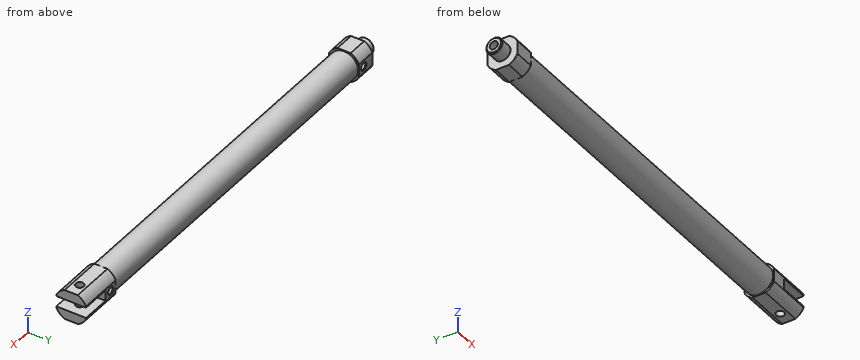
Autodesk Inventor part; units mm, degrees
ref_plane "BODY_N_XY" through (257, 0, 0) normal (0, 0, -1) x (1, 0, 0)
ref_plane "BODY_N_YZ" through (257, 0, 0) normal (1, 0, 0) x (0, -1, 0)
ref_plane "BODY_N_ZX" through (257, 0, 0) normal (0, -1, 0) x (0, 0, -1)
sketch "Sketch_8" plane through (0, 0, 0) normal (0, 0, 1) x (1, 0, 0)
  line L0 (0, 0) -> (-8, 0)
  line L1 (-8, 0) -> (-8, 4.3865)
  line L2 (-8, 4.3865) -> (-7.3865, 5)
  line L3 (-7.3865, 5) -> (0, 5)
  line L4 (0, 5) -> (0, 0)
  line L5 (0, 0) -> (-8, 0)
revolve "Revolution1" add sketch "Sketch_8" angle 360 about axis through (0, 0, 0) along (1, 0, 0)
thread "Thread1"
sketch "Sketch_9" plane through (0, 0, 0) normal (1, 0, 0) x (0, 0, -1)
  line L0 (-9.15, 4.0345) -> (-9.15, -4.0345)
  arc A0 (-9.15, -4.0345) -> (-4.0345, -9.15) centre (0, 0) ccw
  line L1 (-4.0345, -9.15) -> (4.0345, -9.15)
  arc A1 (4.0345, -9.15) -> (9.15, -4.0345) centre (0, 0) ccw
  line L2 (9.15, -4.0345) -> (9.15, 4.0345)
  arc A2 (9.15, 4.0345) -> (4.0345, 9.15) centre (0, 0) ccw
  line L3 (4.0345, 9.15) -> (-4.0345, 9.15)
  arc A3 (-4.0345, 9.15) -> (-9.15, 4.0345) centre (0, 0) ccw
extrude "Extrusion1" add sketch "Sketch_9" along normal blind 12.5
sketch "Sketch_11" plane through (12.5, 0, 0) normal (1, 0, 0) x (0, 0, -1)
  circle A0 centre (0, 0) radius 8.7
extrude "Extrusion2" add sketch "Sketch_11" along normal blind 225
sketch "Sketch_10" plane through (237.5, 0, 0) normal (1, 0, 0) x (0, 0, -1)
  line L0 (-9.15, 4.0345) -> (-9.15, -4.0345)
  arc A0 (-9.15, -4.0345) -> (-4.0345, -9.15) centre (0, 0) ccw
  line L1 (-4.0345, -9.15) -> (4.0345, -9.15)
  arc A1 (4.0345, -9.15) -> (9.15, -4.0345) centre (0, 0) ccw
  line L2 (9.15, -4.0345) -> (9.15, 4.0345)
  arc A2 (9.15, 4.0345) -> (4.0345, 9.15) centre (0, 0) ccw
  line L3 (4.0345, 9.15) -> (-4.0345, 9.15)
  arc A3 (-4.0345, 9.15) -> (-9.15, 4.0345) centre (0, 0) ccw
extrude "Extrusion3" add sketch "Sketch_10" along normal blind 27.5
sketch "Sketch7" plane through (0, 0, 0) normal (0, 0, 1) x (1, 0, 0)
  line L0 (8, 9.15) -> (8, 4.15)
  line L1 (8, 2.9566) -> (5.933, 4.15)
  line L2 (5.933, 4.15) -> (5.933, 8.717)
  line L3 (5.933, 8.717) -> (5.5, 9.15)
  line L4 (5.5, 9.15) -> (8, 9.15)
  line L5 (8, 9.15) -> (8, 2.9566)
revolve "Revolution2" cut sketch "Sketch7" angle 360 about axis through (8, 9.15, 0) along (0, 1, 0)
thread "Thread2"
sketch "Sketch_7" plane through (0, 0, 0) normal (0, 0, 1) x (1, 0, 0)
  line L0 (242, 9.15) -> (242, 4.15)
  line L1 (242, 2.9566) -> (239.933, 4.15)
  line L2 (239.933, 4.15) -> (239.933, 8.717)
  line L3 (239.933, 8.717) -> (239.5, 9.15)
  line L4 (239.5, 9.15) -> (242, 9.15)
  line L5 (242, 9.15) -> (242, 2.9566)
revolve "Revolution3" cut sketch "Sketch_7" angle 360 about axis through (242, 9.15, 0) along (0, 1, 0)
thread "Thread3"
sketch "Sketch_16" plane through (0, 0, 0) normal (0, 0, 1) x (1, 0, 0)
  line L0 (217.5, 0) -> (-8, 0)
  line L1 (-8, 0) -> (-8, 2.5)
  line L2 (-8, 2.5) -> (12.5, 2.5)
  line L3 (12.5, 2.5) -> (12.5, 8)
  line L4 (12.5, 8) -> (217.5, 8)
  line L5 (217.5, 8) -> (217.5, 0)
  line L6 (217.5, 0) -> (-8, 0)
revolve "Revolution4" cut sketch "Sketch_16" angle 360 about axis through (217.5, 0, 0) along (1, 0, 0)
sketch "Sketch_3" plane through (0, 0, 0) normal (0, 1, 0) x (-1, 0, 0)
  line L0 (-247, 3.25) -> (-265, 3.25)
  line L1 (-265, 3.25) -> (-265, -3.25)
  line L2 (-265, -3.25) -> (-247, -3.25)
  line L3 (-247, -3.25) -> (-247, 3.25)
extrude "Extrusion4" cut sketch "Sketch_3" along normal mid plane 18.3
sketch "Sketch_13" plane through (0, 0, 0) normal (0, 0, 1) x (1, 0, 0)
  circle A0 centre (257, 0) radius 2.5
extrude "Extrusion5" cut sketch "Sketch_13" along normal mid plane 18.3
ref_plane "BODY_N_XY" through (257, 0, 0) normal (0, 0, -1) x (1, 0, 0)
ref_plane "BODY_N_YZ" through (257, 0, 0) normal (1, 0, 0) x (0, -1, 0)
ref_plane "BODY_N_ZX" through (257, 0, 0) normal (0, -1, 0) x (0, 0, -1)
ref_plane "BODY_PIN_XY" through (257, 0, 0) normal (-1, 0, 0) x (0, 0, -1)
ref_plane "BODY_PIN_YZ" through (257, 0, 0) normal (0, 0, -1) x (0, -1, 0)
ref_plane "BODY_PIN_ZX" through (257, 0, 0) normal (0, -1, 0) x (-1, 0, 0)
ref_plane "NUT2_XY" through (247, 0, 0) normal (1, 0, 0) x (0, 0, -1)
ref_plane "NUT2_YZ" through (247, 0, 0) normal (0, 0, -1) x (0, 1, 0)
ref_plane "NUT2_ZX" through (247, 0, 0) normal (0, 1, 0) x (1, 0, 0)
ref_plane "SW1_XY" through (17.5, 0, 0) normal (1, 0, 0) x (0, 0, -1)
ref_plane "SW1_YZ" through (17.5, 0, 0) normal (0, 0, -1) x (0, 1, 0)
ref_plane "SW1_ZX" through (17.5, 0, 0) normal (0, 1, 0) x (1, 0, 0)
ref_plane "SW2_XY" through (232.5, 0, 0) normal (-1, 0, 0) x (0, 0, -1)
ref_plane "SW2_YZ" through (232.5, 0, 0) normal (0, 0, -1) x (0, -1, 0)
ref_plane "SW2_ZX" through (232.5, 0, 0) normal (0, -1, 0) x (-1, 0, 0)
ref_plane "SW_R1_XY" through (17.5, -14.15, 0) normal (1, 0, 0) x (0, 0, -1)
ref_plane "SW_R1_YZ" through (17.5, -14.15, 0) normal (0, 0, -1) x (0, 1, 0)
ref_plane "SW_R1_ZX" through (17.5, -14.15, 0) normal (0, 1, 0) x (1, 0, 0)
ref_plane "SW_R2_XY" through (232.5, -14.15, 0) normal (-1, 0, 0) x (0, 0, -1)
ref_plane "SW_R2_YZ" through (232.5, -14.15, 0) normal (0, 0, -1) x (0, -1, 0)
ref_plane "SW_R2_ZX" through (232.5, -14.15, 0) normal (0, -1, 0) x (-1, 0, 0)
ref_plane "body_XY" through (0, 0, 0) normal (1, 0, 0) x (0, 0, -1)
ref_plane "body_YZ" through (0, 0, 0) normal (0, 0, -1) x (0, 1, 0)
ref_plane "body_ZX" through (0, 0, 0) normal (0, 1, 0) x (1, 0, 0)
properties part number "CJ2D16-200Z(1_0)_BODY"
Geometry check sheet. Reference: the model listing, model coordinates, mm. Round coordinates to 2 decimals unless told otherwise and drop trailing zeros. Loops run counter-clockwise (first coordinate to the right, second up) from the corner with the lowest first, then second, coordinate; pieces in that order, holes last. Notation, with made-up numbers: (43.5, 26) -> (89.5, 26) arc R7 cw to (89.5, 37) -> close; hole circle Ø3 at (-4, 52.25). An arc over 180 degrees is marked (long way). Answer as a JSON object with one key per item and string values. Group by question number.
Item 1: Thickness scan on line 1 along X through (y, z) = (2.5, 2.5); line 2 along X through (y, z) = (-5, 7.5); line 3 along X through (y, z) = (2, 4.5). Record the ranges inside material, lowest first.
Item 2: Cross-section at A-A, the plane x = 257. Record the cut outline in (y, z), plus the area to 3 significant figures.
Item 3: Depth check by flat-ended pin: pin 1 Ø6 at (x, z) = (131, -5.5) entering from -Y; pin 2 Ø3 at (y, z) = (-4.5, -6) entering from -X; pin 3 Ø8 at (x, y) = (115, -5.5) entering from +Z; pin 4 Ø3 at (x, y) = (257, 0) entering from +Z. Enter the tip coordinate at first touch or a pass-through.
Item 4: Cross-section at C-C, the plane x = 45. Record the cut outline in (y, z), plus the area to 3 significant figures.
Item 5: Cross-section at B-B, the plane y = 0. Count the separate pieces of the cut face and the enclosed holes in it, plus the area to 3 significant figures.
Determined:
{
 "1": {"line 1": "x = -8 to 12.5, 217.5 to 247", "line 2": "x = 0 to 12.5, 237.5 to 265", "line 3": "x = -7.46 to 12.5, 217.5 to 255.5, 258.5 to 265"},
 "2": {"outline": "(-9.15, -4.03) arc R10 ccw to (-4.03, -9.15) -> (-2.5, -9.15) -> (-2.5, -3.25) -> (-9.15, -3.25) -> close; (-9.15, 3.25) -> (-2.5, 3.25) -> (-2.5, 9.15) -> (-4.03, 9.15) arc R10 ccw to (-9.15, 4.03) -> close; (2.5, -9.15) -> (4.03, -9.15) arc R10 ccw to (9.15, -4.03) -> (9.15, -3.25) -> (2.5, -3.25) -> close; (2.5, 3.25) -> (9.15, 3.25) -> (9.15, 4.03) arc R10 ccw to (4.03, 9.15) -> (2.5, 9.15) -> close", "area": "118 mm²"},
 "3": {"pin 1": "stops at y = -8.33", "pin 2": "stops at x = 0", "pin 3": "stops at z = 8.57", "pin 4": "passes through"},
 "4": {"outline": "circle Ø17.4 at (0, 0); hole circle Ø16 at (0, 0)", "area": "36.7 mm²"},
 "5": {"separate pieces": "3", "enclosed holes": "0", "area": "1,170 mm²"}
}
